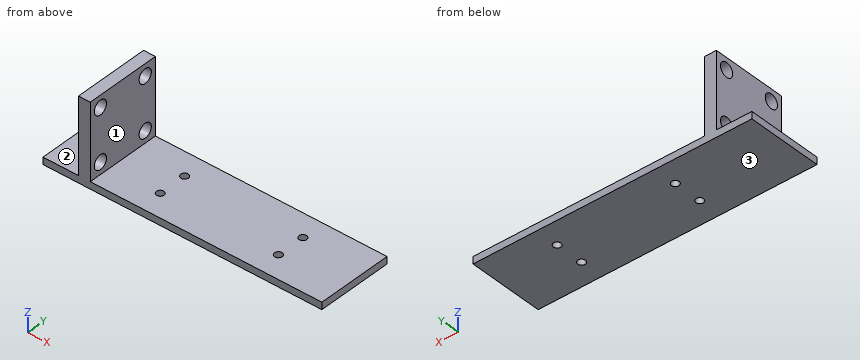
```python
from build123d import *

# Parameters (mm, degrees)
SKETCH_1_W          = 118
SKETCH_1_H          = 32
EXTRUDE_1_DEPTH     = 3
SKETCH_2_R          = 1.62
CUT_EXTRUDE_1_DEPTH = 3
SKETCH_3_W          = 5
SKETCH_3_H          = 32
EXTRUDE_2_DEPTH     = 32
SKETCH_4_R          = 3
CUT_EXTRUDE_2_DEPTH = 32


with BuildPart() as part:
    # 草图1 → 凸台-拉伸1 (new body)
    with BuildSketch(Plane.XY):
        with Locations((-12.281632653, 6.717006803)):
            Rectangle(SKETCH_1_W, SKETCH_1_H)
    extrude(amount=EXTRUDE_1_DEPTH)

    # 草图2 → 切除-拉伸1 (cut)
    with BuildSketch(Plane.XY.offset(3)):
        with Locations((-30.281632653, 12.717006803)):
            Circle(SKETCH_2_R)
        with Locations((-30.281632653, 0.717006803)):
            Circle(SKETCH_2_R)
        with Locations((19.718367347, 12.717006803)):
            Circle(SKETCH_2_R)
        with Locations((19.718367347, 0.717006803)):
            Circle(SKETCH_2_R)
    extrude(amount=-CUT_EXTRUDE_1_DEPTH, mode=Mode.SUBTRACT)

    # 草图3 → 凸台-拉伸2 (add)
    with BuildSketch(Plane.XY.offset(3)):
        with Locations((-53.781632653, 6.717006803)):
            Rectangle(SKETCH_3_W, SKETCH_3_H)
    extrude(amount=EXTRUDE_2_DEPTH)

    # 草图4 → 切除-拉伸2 (cut)
    with BuildSketch(Plane.ZY.offset(71.281632653)):
        with Locations((30, 17.717006803)):
            Circle(SKETCH_4_R)
        with Locations((30, -4.282993197)):
            Circle(SKETCH_4_R)
        with Locations((8, 17.717006803)):
            Circle(SKETCH_4_R)
        with Locations((8, -4.282993197)):
            Circle(SKETCH_4_R)
    extrude(amount=-CUT_EXTRUDE_2_DEPTH, mode=Mode.SUBTRACT)


solid = part.part
```
Model file for the job. Use its own axes, mm. Face numbers are marked on the shaded views. A direction names the side the tool comes from. Coordinates: 2 decimals unless noted, no trailing zeros. Order: outer loops, then holes, each group sorted by start corner. A loop starts at its lowest first (then second) coordinate and runs counter-clockwise, first axis right, second up. Notation, with made-up numbers: (23.5, 60) - (63.5, 60) arc R13 ccw to (63.5, 84) - close; hole circle Ø4 at (30.5, 82.25). An arc over 180 degrees is marked (long way). Return JSON: item names as keys, results as strings. Group by question number.
1) Tool access for the marked faces 1, 2 and 3: list every direction of +Z, -Z, +X, -X, +Y, -Y with a clear straight run to the whole face (end or side of a thin tool).
2) Saw through at D-D, the plane x = 9. Write the cut outline in (y, z), plus the area to 3 significant figures.
3) Saw through at C-C, the plane z = 19.5. Write the cut outline in (x, y), plus the area to 3 significant figures.
4) Saw through at B-B, the plane y = 16. Write the cut outline in (x, z).
5) Probe line 1 (Y direction, x = -54, z = 30); line 2 (Z direction, x = -52, y = 18); line 3 (Z direction, x = -52.5, y = 18.5). List the from-to ranges inside material, lowest first. Write a range as from..to.
6) Saw through at A-A, the plane z = 30. Write the cut outline in (x, y), plus the area to 3 significant figures.
7) Flat gauge pins, fed straight in: P1, Ø16, axis at y = 10.5, z = 22.5, coming from the -X side; P2, Ø3.5, axis at x = 19.72, y = 12.72, coming from the +Z side; P3, Ø9.5, axis at y = -4.28, z = 30, coming from the +X side. Where does each tip first touch, or does it go through?
Values found:
{
 "1": {"face 1": "+Z, +X, +Y, -Y", "face 2": "+Z, -X, +Y, -Y", "face 3": "-Z, +X, -X, +Y, -Y"},
 "2": {"outline": "(-9.28, 0) - (22.72, 0) - (22.72, 3) - (-9.28, 3) - close", "area": "96.0 mm²"},
 "3": {"outline": "(-56.28, -9.28) - (-51.28, -9.28) - (-51.28, 22.72) - (-56.28, 22.72) - close", "area": "160 mm²"},
 "4": {"outline": "(-71.28, 0) - (46.72, 0) - (46.72, 3) - (-51.28, 3) - (-51.28, 5.54) - (-56.28, 5.54) - (-56.28, 3) - (-71.28, 3) - close; (-56.28, 10.46) - (-51.28, 10.46) - (-51.28, 27.54) - (-56.28, 27.54) - close; (-56.28, 32.46) - (-51.28, 32.46) - (-51.28, 35) - (-56.28, 35) - close"},
 "5": {"line 1": "y = -9.28..-7.28, -1.28..14.72, 20.72..22.72", "line 2": "z = 0..5.01, 10.99..27.01, 32.99..35", "line 3": "z = 0..5.1, 10.9..27.1, 32.9..35"},
 "6": {"outline": "(-56.28, -9.28) - (-51.28, -9.28) - (-51.28, -7.28) - (-56.28, -7.28) - close; (-56.28, -1.28) - (-51.28, -1.28) - (-51.28, 14.72) - (-56.28, 14.72) - close; (-56.28, 20.72) - (-51.28, 20.72) - (-51.28, 22.72) - (-56.28, 22.72) - close", "area": "100 mm²"},
 "7": {"P1": "stops at x = -56.28", "P2": "stops at z = 3", "P3": "stops at x = -51.28"}
}
